Work out the finished part from the listing and answer in its coordinate system (mm). Round coordinates to 2 decimals unless told otherwise and drop trailing zeros. Order: outer loops, then holes, each group sorted by start corner. A loop starts at its lowest first (then second) coordinate and runs counter-clockwise, first axis right, second up. Notation, with made-up numbers: (80, -2.75) - (106, -2.75) arc R20 cw to (106, 12.25) - close; hole circle Ø1 at (0.5, 67). An arc over 180 degrees is marked (long way). Use one line per item in the form item = value. Start each with the question number.
Q1. The part is cut by section B-B on z = 0.65. State how many separate pieces and enclosed holes the cut face has, plus the area to 3 significant figures.
Q2. Find the intervals of material crossed by line 1 (Y direction, x = -241.5, z = 0.9); line 2 (Y direction, x = -40, z = 0.85); line 3 (Y direction, x = -7, z = 1.15), in increasing order. Write a range as [from, to].
Q3. The part is cut by section C-C on y = 309.5. Determine the outline of the cut face in (x, z).
Q4. Given P1, Ø3, axis at x = -203, y = 142, coming from the +Z side; P2, Ø0.8, axis at y = 377.5, z = 1, coming from the +X side, each flat-ended and moving along its own axis, determine where each tip first touches the part or whether it passes through.
Q5. The part is cut by section A-A on x = -129. Determine the outline of the cut face in (y, z).
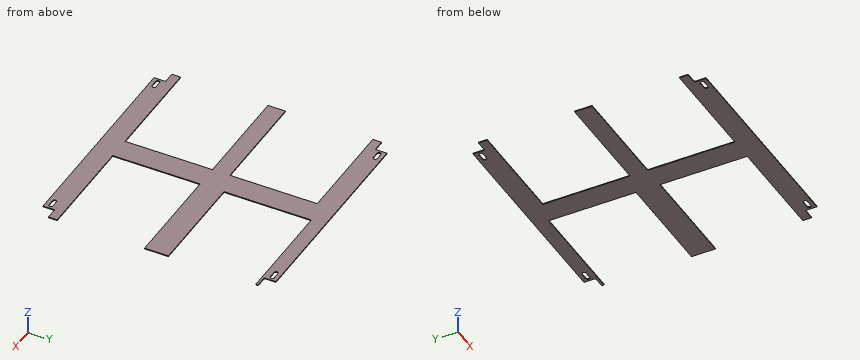
from build123d import *

# Parameters (mm, degrees)
EXTRUDE_1_DEPTH = 1.5


with BuildPart() as part:
    # 草图1 → 凸台-拉伸1 (new body)
    with BuildSketch(Plane.XY):
        Polygon((-10, 366), (-160, 366), (-160, 216), (-10, 216), (20, 216), (20, 175), (-10, 175), (-160, 175), (-160, 25), (-10, 25), (20, 25), (20, 10), (0, 10), (0, -10), (-360, -10), (-360, 10), (-380, 10), (-380, 25), (-350, 25), (-200, 25), (-200, 175), (-350, 175), (-380, 175), (-380, 205), (-350, 205), (-200, 205), (-200, 355), (-350, 355), (-380, 355), (-380, 370), (-360, 370), (-360, 390), (0, 390), (0, 370), (20, 370), (20, 366), align=None)
        with BuildLine():
            Line((-353, -3.25), (-341, -3.25))
            ThreePointArc((-341, -3.25), (-337.75, 0), (-341, 3.25))
            Line((-341, 3.25), (-353, 3.25))
            ThreePointArc((-353, 3.25), (-356.25, 0), (-353, -3.25))
        make_face(mode=Mode.SUBTRACT)
        with BuildLine():
            Line((-19, -3.25), (-7, -3.25))
            ThreePointArc((-7, -3.25), (-3.75, 0), (-7, 3.25))
            Line((-7, 3.25), (-19, 3.25))
            ThreePointArc((-19, 3.25), (-22.25, 0), (-19, -3.25))
        make_face(mode=Mode.SUBTRACT)
        with BuildLine():
            Line((-19, 376.75), (-7, 376.75))
            ThreePointArc((-7, 376.75), (-3.75, 380), (-7, 383.25))
            Line((-7, 383.25), (-19, 383.25))
            ThreePointArc((-19, 383.25), (-22.25, 380), (-19, 376.75))
        make_face(mode=Mode.SUBTRACT)
        with BuildLine():
            Line((-353, 376.75), (-341, 376.75))
            ThreePointArc((-341, 376.75), (-337.75, 380), (-341, 383.25))
            Line((-341, 383.25), (-353, 383.25))
            ThreePointArc((-353, 383.25), (-356.25, 380), (-353, 376.75))
        make_face(mode=Mode.SUBTRACT)
    extrude(amount=EXTRUDE_1_DEPTH)


solid = part.part
Found:
q1.separate_pieces = 1
q1.enclosed_holes = 4
q1.area = 50,000 mm²
q2.line_1 = [-10, 25], [175, 205], [355, 390]
q2.line_2 = [-10, 25], [175, 216], [366, 390]
q2.line_3 = [-10, -3.25], [3.25, 25], [175, 216], [366, 376.75], [383.25, 390]
q3.outline = (-200, 0) - (-160, 0) - (-160, 1.5) - (-200, 1.5) - close
q4.P1 = through
q4.P2 = 0
q5.outline = (-10, 0) - (25, 0) - (25, 1.5) - (-10, 1.5) - close; (175, 0) - (216, 0) - (216, 1.5) - (175, 1.5) - close; (366, 0) - (390, 0) - (390, 1.5) - (366, 1.5) - close
